Input: part model. Units: mm. Frame: model coordinates. A direction names the side the tool comes from. Round coordinates to 2 decimals unless told otherwise and drop trailing zeros. Loops run counter-clockwise (first coordinate to the right, second up) from the corner with the lowest first, then second, coordinate; pieces in that order, holes last. Notation, with made-up numbers: (70.5, 65.25) -> (109.5, 65.25) arc R14 cw to (109.5, 90.25) -> close; hole circle Ø1 at (-20, 38.25). An arc over 180 degrees is marked (long way). One line per question, with ' | ' between items. Start each with the question number.
Q1. Cut plane B-B on x = 5. Return loops of the section in (y, z).
Q2. Cut plane A-A on x = 52.5. Return loops of the section in (y, z).
Q3. Contact query for flat-ended pins moving along their axis: P1, Ø1, axis at x = 37, z = 24.5, coming from the +Y side; P2, Ø5, axis at y = 6.5, z = 23.5, coming from the +X side; P3, Ø1.8, axis at x = 30.5, y = 5, coming from the +Z side; P4, Ø3, axis at x = 46, y = 5.5, coming from the +Z side. Output: stop coordinate, or through.
Q4. Cut plane C-C on z = 4. Return loops of the section in (x, y), and give its area (3 significant figures).
Q5. Access query for faces 5 (the face through (36, 5, 18)), 6 (the face through (11, 5, 28.5)), 7 (the face through (23.606, 4.93, 35.86)). Directions: +Z, -Z, +X, -X, +Y, -Y. A direction counts if a zero-diameter tool reaches every point of the face in a straight line with its end or side. Return the directions, or none.
Q6. Material intervals for L1, parallel to Y at x = 5, z = 1; L2, parallel to Z at x = 54, y = 8.5; L3, parallel to X at y = 4.75, z = 30, sorted ascending.
Q7. Mould query, pull axis X, two halves, no side actions, for faces 1 (the face through (10, 5, 35)), 2 (the face through (60, 5, 32)), 3 (the face through (0.9, 9.14, 3.2)), 4 (the face through (30, 5, 20)). Classes: pulls with the +X half, pulls with the -X half, needs draft (parallel to the pull), parting line crosses it, or undercut.
Q8. Cut plane D-D on y = 5. State how many separate pieces and enclosed holes the cut face has, and give its area (3 significant figures).
from build123d import *

# Parameters (mm, degrees)
SKETCH1_W               = 60
SKETCH1_H               = 35
BOSS_EXTRUDE1_DEPTH     = 10
SKETCH2_W               = 22
SKETCH2_H               = 10
CUT_EXTRUDE1_DEPTH      = 24
SKETCH3_W               = 22
SKETCH3_H               = 10
CUT_EXTRUDE2_DEPTH      = 25
SKETCH5_R               = 1.45
CUT_EXTRUDE4_DEPTH      = 71.178344238
FILLET1_R               = 3
FILLET2_R               = 3
SKETCH7_W               = 11
SKETCH7_H               = 10
BOSS_EXTRUDE2_DEPTH     = 3
CUT_EXTRUDE5_DEPTH      = 3
CUT_EXTRUDE5_DEPTH_BACK = 15
SKETCH6_R               = 1.5
FILLET3_R               = 4


with BuildPart() as part:
    # Sketch1 → Boss-Extrude1 (new body)
    with BuildSketch(Plane(origin=(0, 0, 0), x_dir=(1, 0, 0), z_dir=(0, 1, 0))):
        with Locations((30, -17.5)):
            Rectangle(SKETCH1_W, SKETCH1_H)
    extrude(amount=BOSS_EXTRUDE1_DEPTH)

    # Sketch2 → Cut-Extrude1 (cut)
    with BuildSketch(Plane(origin=(60, 0, 0), x_dir=(0, 0, -1), z_dir=(1, 0, 0))):
        with Locations((-17.5, 5)):
            Rectangle(SKETCH2_W, SKETCH2_H)
    extrude(amount=-CUT_EXTRUDE1_DEPTH, mode=Mode.SUBTRACT)

    # Sketch3 → Cut-Extrude2 (cut)
    with BuildSketch(Plane.ZY):
        with Locations((17.5, 5)):
            Rectangle(SKETCH3_W, SKETCH3_H)
    extrude(amount=-CUT_EXTRUDE2_DEPTH, mode=Mode.SUBTRACT)

    # Sketch5 → Cut-Extrude4 (cut, through all)
    with BuildSketch(Plane.XY.offset(35)):
        with Locations((5, 5)):
            Circle(SKETCH5_R)
        with Locations((55, 5)):
            Circle(SKETCH5_R)
    extrude(amount=-CUT_EXTRUDE4_DEPTH, mode=Mode.SUBTRACT)

    # Fillet1
    fillet1_edges = [part.edges().sort_by_distance(p)[0] for p in [
        (60, 10, 31.75),
        (60, 0, 3.25),
        (60, 10, 3.25),
        (0, 0, 31.75),
        (0, 10, 31.75),
        (0, 10, 3.25),
        (60, 0, 31.75),
        (0, 0, 3.25),
    ]]
    fillet(fillet1_edges, radius=FILLET1_R)

    # Fillet2
    fillet2_edges = [part.edges().sort_by_distance(p)[0] for p in [
        (36, 5, 28.5),
        (36, 5, 6.5),
        (25, 5, 6.5),
        (25, 5, 28.5),
    ]]
    fillet(fillet2_edges, radius=FILLET2_R)

    # Sketch7 → Boss-Extrude2 (add)
    with BuildSketch(Plane.XY.offset(35)):
        with Locations((30.5, 5)):
            Rectangle(SKETCH7_W, SKETCH7_H)
    extrude(amount=BOSS_EXTRUDE2_DEPTH)

    # Sketch6 → Cut-Extrude5 (cut, two sides: drawn at the far end of the back side and taken through both)
    with BuildSketch(Plane.XY.offset(35).offset(-CUT_EXTRUDE5_DEPTH_BACK)):
        with Locations((30.5, 5)):
            Circle(SKETCH6_R)
    extrude(amount=CUT_EXTRUDE5_DEPTH + CUT_EXTRUDE5_DEPTH_BACK, mode=Mode.SUBTRACT)

    # Fillet3
    # the kernel refuses this fillet: 4 mm, written as the material it adds along each edge
    with BuildSketch(Plane(origin=(36, 10, 35), x_dir=(0, 0, 1), z_dir=(0, -1, 0))) as fillet3_piece_1:
        with BuildLine():
            CenterArc((4, -3.872983346), FILLET3_R, 104.477512186, 75.522487814)
            Line((0, -3.872983346), (-0.08, -3.872983346))
            Line((-0.08, -3.872983346), (-0.08, 0))
            Line((-0.08, 0), (0, 0.08))
            ThreePointArc((0, 0.08), (1.5, 0.08), (2.98, 0.077459667))
            Line((2.98, 0.077459667), (3, 0))
        make_face()
    extrude(amount=10)
    with BuildSketch(Plane(origin=(25, 0, 35), x_dir=(-1, 0, 0), z_dir=(0, 1, 0))) as fillet3_piece_2:
        with BuildLine():
            CenterArc((3.872983346, 4), FILLET3_R, 194.477512186, 75.522487814)
            Line((0, 3), (-0.077459667, 2.98))
            ThreePointArc((-0.077459667, 2.98), (-0.08, 1.5), (-0.08, 0))
            Line((-0.08, 0), (0, -0.08))
            Line((0, -0.08), (3.872983346, -0.08))
            Line((3.872983346, -0.08), (3.872983346, 0))
        make_face()
    extrude(amount=10)


solid = part.part
Results:
1) outline: (0, 0) -> (3.55, 0) -> (3.55, 6.5) -> (0, 6.5) -> close; (0, 28.5) -> (3.55, 28.5) -> (3.55, 35) -> (0, 35) -> close; (6.45, 0) -> (10, 0) -> (10, 6.5) -> (6.45, 6.5) -> close; (6.45, 28.5) -> (10, 28.5) -> (10, 35) -> (6.45, 35) -> close
2) outline: (0, 0) -> (10, 0) -> (10, 6.5) -> (0, 6.5) -> close; (0, 28.5) -> (10, 28.5) -> (10, 35) -> (0, 35) -> close
3) P1: through | P2: x = 36.04 | P3: z = 20 | P4: z = 35
4) outline: (0, 3) arc R3 ccw to (3, 0) -> (57, 0) arc R3 ccw to (60, 3) -> (60, 7) arc R3 ccw to (57, 10) -> (3, 10) arc R3 ccw to (0, 7) -> close; hole circle Ø2.9 at (5, 5); hole circle Ø2.9 at (55, 5) | area: 579 mm^2
5) face 5: +X, +Y, -Y | face 6: -X, +Y, -Y | face 7: +Z, -X, +Y, -Y
6) L1: 0 to 3.55, 6.45 to 10 | L2: 0 to 6.5, 28.5 to 35 | L3: 0 to 3.57, 6.43 to 29.02, 31.98 to 53.57, 56.43 to 60
7) face 1: needs draft | face 2: pulls with the +X half | face 3: pulls with the -X half | face 4: undercut
8) separate pieces: 5 | enclosed holes: 0 | area: 939 mm^2
